The listing builds one solid part. Answer for the finished solid, in the listing's coordinates (mm). Round coordinates to 2 decimals unless told otherwise and drop trailing zeros. Write each loop counter-clockwise with the first axis right and the second up, starting at its lowest first coordinate (ties: lowest second). Pieces come first, ordered by that corner, then holes. Notation, with made-up numbers: (14, 85.25) - (29, 85.25) arc R14 ccw to (29, 111.25) - close; hole circle Ø11 at (29.25, -2). An arc over 180 degrees is marked (long way). Use a Markdown table: item, result. Add a question column.
1) Each of these flat-tipped pins is pushed along its axis until it touches: P1, Ø4, axis at x = -21.5, z = 28.5, coming from the -Y side; P2, Ø3, axis at x = 9.5, y = 2.5, coming from the -Z side; P3, Ø3, axis at x = 26, y = 3.5, coming from the +Z side. Where does it stop, or does it pass through?
2) A cutting plane is placed at D-D (x = -52.5). Give the vertices of the cut face in (y, z).
3) Find the intervals of material crossed by probe 1 along Z at (x, y) = (-22.5, 4.6); probe 2 along Z at (x, y) = (22.5, 1.45); probe 3 along X at (y, z) = (4.1, 5), in increasing order. Write a range as from..to.
4) A cutting plane is placed at C-C (y = 2.3). State how many separate pieces and enclosed holes the cut face has, then the cut area to 3 significant figures.
5) A cutting plane is placed at B-B (x = 43). Give the vertices of the cut face in (y, z).
6) A cutting plane is placed at A-A (z = -44). Give the vertices of the cut face in (x, y).
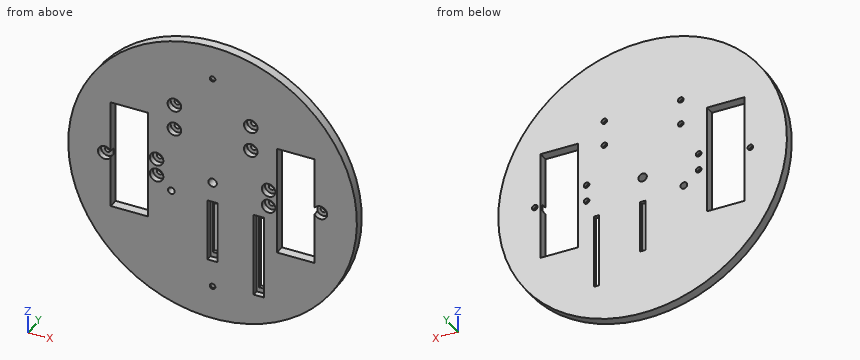
```python
from build123d import *

# Parameters (mm, degrees)
SKETCH1_R                      = 85
SKETCH1_R_2                    = 2.5
SKETCH1_R_3                    = 2
SKETCH1_W                      = 22
SKETCH1_H                      = 65
BOSS_EXTRUDE1_DEPTH            = 5.588
CBORE_FOR_M3_SHCS1_D           = 3.3
CBORE_FOR_M3_SHCS1_CBORE_D     = 8
CBORE_FOR_M3_SHCS1_CBORE_DEPTH = 3.5
CBORE_FOR_M3_SHCS2_D           = 3.3
CBORE_FOR_M3_SHCS2_CBORE_D     = 8
CBORE_FOR_M3_SHCS2_CBORE_DEPTH = 3.5
SKETCH16_R                     = 1.65
CUT_EXTRUDE1_DEPTH             = 1
SKETCH17_W                     = 3.2
SKETCH17_H                     = 44
SKETCH17_H_2                   = 31
CUT_EXTRUDE2_DEPTH             = 121.337964683
SKETCH20_W                     = 6
SKETCH20_H                     = 50
SKETCH20_H_2                   = 37
CUT_EXTRUDE6_DEPTH             = 3.5


with BuildPart() as part:
    # Sketch1 → Boss-Extrude1 (new body)
    with BuildSketch(Plane(origin=(0, 0, 0), x_dir=(1, 0, 0), z_dir=(0, 1, 0))):
        with Locations(Location((0, 0, 0), (0, 0, 270))):
            Circle(SKETCH1_R)
        with Locations(Location((0, 0, 0), (0, 0, 270))):
            Circle(SKETCH1_R_2, mode=Mode.SUBTRACT)
        with Locations(Location((-24.317199098, 12.25, 0), (0, 0, 270))):
            Circle(SKETCH1_R_3, mode=Mode.SUBTRACT)
        with Locations((-49, 0)):
            Rectangle(SKETCH1_W, SKETCH1_H, mode=Mode.SUBTRACT)
        with Locations((49, 0)):
            Rectangle(SKETCH1_W, SKETCH1_H, mode=Mode.SUBTRACT)
    extrude(amount=BOSS_EXTRUDE1_DEPTH)

    # CBORE for M3 SHCS1 (through all)
    with Locations(Plane(origin=(0, 0, 0), x_dir=(-1, 0, 0), z_dir=(0, -1, 0))):
        with Locations((-33, 5), (-33, -5), (33, 5), (33, -5), (-63.5, 0), (63.5, 0)):
            CounterBoreHole(CBORE_FOR_M3_SHCS1_D / 2, CBORE_FOR_M3_SHCS1_CBORE_D / 2, CBORE_FOR_M3_SHCS1_CBORE_DEPTH)

    # CBORE for M3 SHCS2 (through all)
    with Locations(Plane(origin=(0, 0, 0), x_dir=(-1, 0, 0), z_dir=(0, -1, 0))):
        with Locations((22.5, -26.887097638), (-22.5, -26.887097638), (22.5, -41.887097638), (-22.5, -41.887097638)):
            CounterBoreHole(CBORE_FOR_M3_SHCS2_D / 2, CBORE_FOR_M3_SHCS2_CBORE_D / 2, CBORE_FOR_M3_SHCS2_CBORE_DEPTH)

    # Sketch16 → Cut-Extrude1 (cut)
    with BuildSketch(Plane.XZ):
        with Locations(Location((0, -65, 0), (0, 0, 270))):
            Circle(SKETCH16_R)
        with Locations(Location((0, 65, 0), (0, 0, 90))):
            Circle(SKETCH16_R)
    extrude(amount=-CUT_EXTRUDE1_DEPTH, mode=Mode.SUBTRACT)

    # Sketch17 → Cut-Extrude2 (cut, through all)
    with BuildSketch(Plane.XZ):
        with Locations((27.15, -38)):
            Rectangle(SKETCH17_W, SKETCH17_H)
        with Locations((0, -30.5)):
            Rectangle(SKETCH17_W, SKETCH17_H_2)
    extrude(amount=-CUT_EXTRUDE2_DEPTH, mode=Mode.SUBTRACT)

    # Sketch20 → Cut-Extrude6 (cut)
    with BuildSketch(Plane(origin=(0, 0, 0), x_dir=(-1, 0, 0), z_dir=(0, 1, 0))):
        with Locations((-27.15, -38)):
            Rectangle(SKETCH20_W, SKETCH20_H)
        with Locations((0, -30.5)):
            Rectangle(SKETCH20_W, SKETCH20_H_2)
    extrude(amount=CUT_EXTRUDE6_DEPTH, mode=Mode.SUBTRACT)


solid = part.part
```
Entries:
| question | item | result |
|---|---|---|
| 1 | P1 | stops at y = 3.5 |
| 1 | P2 | stops at z = -84.62 |
| 1 | P3 | stops at z = 81.39 |
| 2 | outline | (0, -66.85) - (5.59, -66.85) - (5.59, -32.5) - (0, -32.5) - close; (0, 32.5) - (5.59, 32.5) - (5.59, 66.85) - (0, 66.85) - close |
| 3 | probe 1 | z = -81.97..-13.09, -11.41..25.24, 28.54..40.24, 43.54..81.97 |
| 3 | probe 2 | z = -81.97..22.89, 30.89..37.89, 45.89..81.97 |
| 3 | probe 3 | x = -84.85..-60, -38..-34.65, -31.35..31.35, 34.65..38, 60..84.85 |
| 4 | separate pieces | 1 |
| 4 | enclosed holes | 14 |
| 4 | area | 18,800 mm² |
| 5 | outline | (0, -73.32) - (5.59, -73.32) - (5.59, -32.5) - (0, -32.5) - close; (0, 32.5) - (5.59, 32.5) - (5.59, 73.32) - (0, 73.32) - close |
| 6 | outline | (-72.73, 0) - (-3, 0) - (-3, 3.5) - (-1.6, 3.5) - (-1.6, 5.59) - (-72.73, 5.59) - close; (1.6, 3.5) - (3, 3.5) - (3, 0) - (24.15, 0) - (24.15, 3.5) - (25.55, 3.5) - (25.55, 5.59) - (1.6, 5.59) - close; (28.75, 3.5) - (30.15, 3.5) - (30.15, 0) - (72.73, 0) - (72.73, 5.59) - (28.75, 5.59) - close |
